Source: CAD feature listing. Evaluate the final solid. Frame: model axes, mm. Face numbers are marked on the shaded views. A direction names the side the tool comes from. Give positions to 0.01 mm unless a question says otherwise; leave off trailing zeros. Write each loop counter-clockwise with the first axis right and the second up, starting at its lowest first coordinate (ties: lowest second). Pieces come first, ordered by that corner, then holes. Notation, with made-up numbers: (81, 69.5) -> (92, 69.5) arc R13 ccw to (92, 91.5) -> close; hole circle Ø1 at (29.5, -31). An arc over 180 degrees is marked (long way). Answer as a JSON object with one key per item and string values. Group by question number.
Item 1: Ray query, probe 1 along X at (y, z) = (38, -1); probe 2 along Z at (x, y) = (13, 3); probe 3 along Z at (x, y) = (38, 1). Return the intervals inside material, ascending. Write a range as from..to.
Item 2: Section query D-D on x = 31.5. Return the cut outline in (y, z) (3 decimals), plus the area to 3 significant figures.
Item 3: Section query B-B on x = 12.7. Return the cut outline in (y, z) (3 decimals), plus the area to 3 significant figures.
Item 4: Section query A-A on y = 38.1. Return the cut outline in (x, z) (3 decimals).
Item 5: Access query for the marked faces 1 and 2. Directions: +Z, -Z, +X, -X, +Y, -Y. A direction counts if a zero-diameter tool reaches every point of the face in a straight line with its end or side. Return the directions, or none.
Item 6: Section query C-C on z = -38.1. Return the cut outline in (x, y) (3 decimals).
Item 7: First-contact query: pin 1 Ø1 at (x, y) = (45.5, 23) entering from -Z (3 decimals); pin 2 Ø4 at (x, y) = (38.1, 15.875) entering from -Z; pin 3 Ø20.5 at (x, z) = (19, -35.5) entering from +Y (3 decimals); pin 4 Ø12 at (x, y) = (12.5, 11) entering from -Z. Flat tips, straight axial feed; report the tip coordinate or a pass-through.
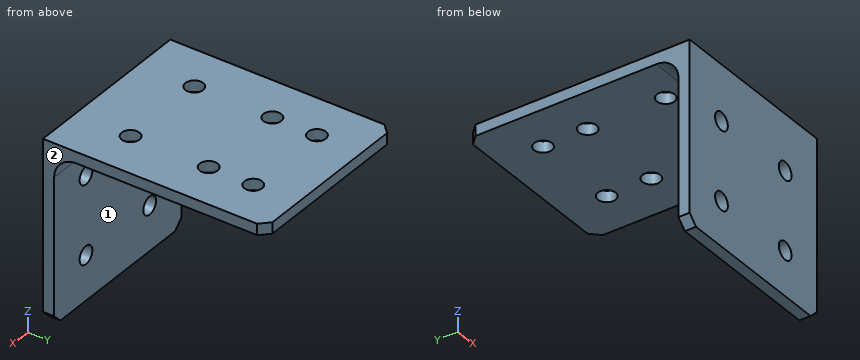
from build123d import *

# Parameters (mm, degrees)
BOSS_EXTRUDE1_DEPTH = 50.8
SKETCH2_R           = 2.54
CUT_EXTRUDE1_DEPTH  = 96.882897328
SKETCH3_R           = 2.54
CUT_EXTRUDE2_DEPTH  = 96.882897328
FILLET1_R           = 6.35
CHAMFER1_SIZE       = 2.54


with BuildPart() as part:
    # Sketch1 → Boss-Extrude1 (new body)
    with BuildSketch(Plane(origin=(0, 0, 0), x_dir=(0, 0, -1), z_dir=(1, 0, 0))):
        Polygon((0, 0), (0, 63.5), (3.175, 63.5), (3.175, 3.175), (50.8, 3.175), (50.8, 0), align=None)
    extrude(amount=BOSS_EXTRUDE1_DEPTH)

    # Sketch2 → Cut-Extrude1 (cut, through all)
    with BuildSketch(Plane.XY):
        with Locations((12.7, 38.1)):
            Circle(SKETCH2_R)
        with Locations((12.7, 15.875)):
            Circle(SKETCH2_R)
        with Locations((12.7, 50.8)):
            Circle(SKETCH2_R)
        with Locations(Location((38.1, 50.8, 0), (0, 0, 270))):
            Circle(SKETCH2_R)
        with Locations(Location((38.1, 15.875, 0), (0, 0, 270))):
            Circle(SKETCH2_R)
        with Locations(Location((38.1, 38.1, 0), (0, 0, 270))):
            Circle(SKETCH2_R)
    extrude(amount=-CUT_EXTRUDE1_DEPTH, mode=Mode.SUBTRACT)

    # Sketch3 → Cut-Extrude2 (cut, through all)
    with BuildSketch(Plane.XZ):
        with Locations(Location((38.1, -38.1, 0), (0, 0, 270))):
            Circle(SKETCH3_R)
        with Locations(Location((38.1, -15.875, 0), (0, 0, 270))):
            Circle(SKETCH3_R)
        with Locations(Location((12.7, -38.1, 0), (0, 0, 270))):
            Circle(SKETCH3_R)
        with Locations(Location((12.7, -15.875, 0), (0, 0, 270))):
            Circle(SKETCH3_R)
    extrude(amount=-CUT_EXTRUDE2_DEPTH, mode=Mode.SUBTRACT)

    # Fillet1
    fillet1_edges = [part.edges().sort_by_distance(p)[0] for p in [
        (25.4, 3.175, -3.175),
    ]]
    fillet(fillet1_edges, radius=FILLET1_R)

    # Chamfer1
    chamfer1_edges = [part.edges().sort_by_distance(p)[0] for p in [
        (50.8, 63.5, -1.5875),
        (0, 63.5, -1.5875),
        (0, 1.5875, -50.8),
        (50.8, 1.5875, -50.8),
    ]]
    chamfer(chamfer1_edges, length=CHAMFER1_SIZE)


solid = part.part
Worked answers:
{
 "1": {"probe 1": "0..10.16, 15.24..35.56, 40.64..50.8", "probe 2": "-50.8..-40.62, -35.58..-18.4, -13.35..0", "probe 3": "-50.8..-40.64, -35.56..-18.41, -13.34..0"},
 "2": {"outline": "(0, -50.8) -> (3.175, -50.8) -> (3.175, -9.525) arc R6.35 cw to (9.525, -3.175) -> (63.5, -3.175) -> (63.5, 0) -> (0, 0) -> close", "area": "361 mm^2"},
 "3": {"outline": "(0, -50.8) -> (3.175, -50.8) -> (3.175, -40.64) -> (0, -40.64) -> close; (0, -35.56) -> (3.175, -35.56) -> (3.175, -18.415) -> (0, -18.415) -> close; (0, -13.335) -> (3.175, -13.335) -> (3.175, -9.525) arc R6.35 cw to (9.525, -3.175) -> (13.335, -3.175) -> (13.335, 0) -> (0, 0) -> close; (18.415, -3.175) -> (35.56, -3.175) -> (35.56, 0) -> (18.415, 0) -> close; (40.64, -3.175) -> (48.26, -3.175) -> (48.26, 0) -> (40.64, 0) -> close; (53.34, -3.175) -> (63.5, -3.175) -> (63.5, 0) -> (53.34, 0) -> close", "area": "281 mm^2"},
 "4": {"outline": "(0, -3.175) -> (10.16, -3.175) -> (10.16, 0) -> (0, 0) -> close; (15.24, -3.175) -> (35.56, -3.175) -> (35.56, 0) -> (15.24, 0) -> close; (40.64, -3.175) -> (50.8, -3.175) -> (50.8, 0) -> (40.64, 0) -> close"},
 "5": {"face 1": "-Z, +X, -X, +Y", "face 2": "+Z, -Z, +X, +Y, -Y"},
 "6": {"outline": "(0, 0) -> (10.16, 0) -> (10.16, 3.175) -> (0, 3.175) -> close; (15.24, 0) -> (35.56, 0) -> (35.56, 3.175) -> (15.24, 3.175) -> close; (40.64, 0) -> (50.8, 0) -> (50.8, 3.175) -> (40.64, 3.175) -> close"},
 "7": {"pin 1": "z = -3.175", "pin 2": "through", "pin 3": "y = 3.175", "pin 4": "z = -5.07"}
}
